Can you work these out from the model? Positions are in its coordinate system, mm. Round coordinates to 2 decimals unless told otherwise and drop trailing zeros. Order: outer loops, then holes, each group sorted by start corner. A loop starts at its lowest first (then second) coordinate and runs counter-clockwise, first axis right, second up. Notation, with made-up numbers: M 89.25,18 L 148.25,18 A22 ccw 148.25,43 Z; hole C 47.25,-26 d4. An arc over 180 degrees is marked long. Answer as a JSON object with one key per item and string values. Group by question number.
Autodesk Fusion 360 part; units mm, degrees
sketch "Sketch1" plane through (0, 0, 0) normal (0, 0, 1) x (1, 0, 0)
  line L0 (0, 0) -> (65, 0)
  line L1 (65, 0) -> (65, 19)
  line L2 (65, 19) -> (0, 19)
  line L3 (0, 19) -> (0, 0)
  circle A0 centre (3.5, 15.5) radius 1.5
  line L4 (32.5, 19) -> (32.5, 0) construction
  line L5 (65, 9.5) -> (0, 9.5) construction
  circle A1 centre (61.5, 15.5) radius 1.5
  circle A2 centre (3.5, 3.5) radius 1.5
  circle A3 centre (61.5, 3.5) radius 1.5
  line L6 (57.77, 13.2) -> (7.23, 13.2)
  line L7 (7.23, 13.2) -> (7.23, 18.2)
  line L8 (7.23, 18.2) -> (57.77, 18.2)
  line L9 (57.77, 18.2) -> (57.77, 13.2)
  line L10 (57.77, 13.2) -> (7.23, 18.2) construction
  line L11 (7.23, 13.2) -> (57.77, 18.2) construction
  line L12 (7.23, 0.8) -> (57.77, 0.8)
  line L13 (57.77, 0.8) -> (57.77, 5.8)
  line L14 (57.77, 5.8) -> (7.23, 5.8)
  line L15 (7.23, 5.8) -> (7.23, 0.8)
  line L16 (57.77, 3.3) -> (7.23, 3.3) construction
  point P0 (32.5, 15.7)
  dimension "d1" = 65
  dimension "d2" = 19
  dimension "d3" = 3
  dimension "d4" = 3.5
  dimension "d5" = 3.5
  dimension "d6" = 50.54
  dimension "d7" = 5
  dimension "d8" = 0.8
extrude "Extrude1" add sketch "Sketch1" along normal blind 0.8 contours L0 L1 L2 L3 | L6 L7 L8 L9 | L12 L13 L14 L15
fillet "Fillet1" radius 3 4 edges at (65, 19, 0.4) (0, 0, 0.4) (65, 0, 0.4) (0, 19, 0.4)
extrude "Extrude2" add sketch "Sketch1" along normal blind 0.4 from surface at 0.8 contours L6 L7 L8 L9 | L12 L13 L14 L15
extrude "Extrude3" add sketch "Sketch1" against normal blind 0.4 contours L6 L7 L8 L9 | L12 L13 L14 L15
Item 1: I need wall thicknesses on line 1 (Y direction, x = 61.5, z = 0.3); line 2 (X direction, y = 16, z = 0.55); line 3 (Z direction, x = 14, y = 10.25). Which ranges of each line are inside material? Lowest first, please.
Item 2: Suppose I cut it at D-D, the plane y = 8. Write out the boundary of the cut face in (x, z).
Item 3: I'm going to push flat-ended pins straight in: pin 1 Ø4 at (x, y) = (3.5, 3.5) entering from +Z; pin 2 Ø1.8 at (x, y) = (3.5, 15.5) entering from +Z; pin 3 Ø3 at (x, y) = (40, 7.5) entering from -Z. Where does each tip first touch, or does it pass through?
Item 4: If we mould it in two halves opening along X, with no side actions, what happens to faces 1 (the face through (32, 10, 0)), 2 (the face through (62.93, 3.05, 0.39)), 3 (the face through (64.1, 0.86, 0.41))? For each: +X half, -X half, draft (parallel to the pull), parting line (faces both ways), or undercut.
Item 5: Suppose I cut it at C-C, the plane x = 4. Write out the boundary of the cut face in (y, z), and give its area (3 significant figures).
Item 6: Suppose I cut it at B-B, the plane x = 31.5. Write out the boundary of the cut face in (y, z), and give its area (3 significant figures).
Item 7: Suppose I cut it at A-A, the plane z = 0.5. Write out the boundary of the cut face in (x, y), and give its area (3 significant figures).
Computed:
{
 "1": {"line 1": "y = 0 to 2, 5 to 14, 17 to 19", "line 2": "x = 0 to 2.09, 4.91 to 60.09, 62.91 to 65", "line 3": "z = 0 to 0.8"},
 "2": {"outline": "M 0,0 L 65,0 L 65,0.8 L 0,0.8 Z"},
 "3": {"pin 1": "stops at z = 0.8", "pin 2": "passes through", "pin 3": "stops at z = 0"},
 "4": {"face 1": "draft", "face 2": "undercut", "face 3": "+X half"},
 "5": {"outline": "M 0,0 L 2.09,0 L 2.09,0.8 L 0,0.8 Z; M 4.91,0 L 14.09,0 L 14.09,0.8 L 4.91,0.8 Z; M 16.91,0 L 19,0 L 19,0.8 L 16.91,0.8 Z", "area": "10.7 mm^2"},
 "6": {"outline": "M 0,0 L 0.8,0 L 0.8,-0.4 L 5.8,-0.4 L 5.8,0 L 13.2,0 L 13.2,-0.4 L 18.2,-0.4 L 18.2,0 L 19,0 L 19,0.8 L 18.2,0.8 L 18.2,1.2 L 13.2,1.2 L 13.2,0.8 L 5.8,0.8 L 5.8,1.2 L 0.8,1.2 L 0.8,0.8 L 0,0.8 Z", "area": "23.2 mm^2"},
 "7": {"outline": "M 0,3 A3 ccw 3,0 L 62,0 A3 ccw 65,3 L 65,16 A3 ccw 62,19 L 3,19 A3 ccw 0,16 Z; hole C 3.5,3.5 d3; hole C 3.5,15.5 d3; hole C 61.5,3.5 d3; hole C 61.5,15.5 d3", "area": "1,200 mm^2"}
}
